from build123d import *

# Parameters (mm, degrees)
SKETCH1_W           = 170
SKETCH1_H           = 16
BOSS_EXTRUDE1_DEPTH = 2
SKETCH2_W           = 25
SKETCH2_H           = 4
CUT_EXTRUDE1_DEPTH  = 86.469292731
FILLET1_R           = 5


with BuildPart() as part:
    # Sketch1 → Boss-Extrude1 (new, symmetric)
    with BuildSketch(Plane(origin=(0, 0, 0), x_dir=(1, 0, 0), z_dir=(0, 1, 0))):
        Rectangle(SKETCH1_W, SKETCH1_H)
    extrude(amount=BOSS_EXTRUDE1_DEPTH, both=True)

    # Sketch2 → Cut-Extrude1 (cut, through all)
    with BuildSketch(Plane(origin=(0, 2, 0), x_dir=(1, 0, 0), z_dir=(0, 1, 0))):
        with Locations((47.5, 6)):
            Rectangle(SKETCH2_W, SKETCH2_H)
        with Locations((-2.5, 6)):
            Rectangle(SKETCH2_W, SKETCH2_H)
        with Locations((-52.5, 6)):
            Rectangle(SKETCH2_W, SKETCH2_H)
        with Locations((-102.5, 6)):
            Rectangle(SKETCH2_W, SKETCH2_H)
        with Locations((-152.5, 6)):
            Rectangle(SKETCH2_W, SKETCH2_H)
        with Locations((-202.5, 6)):
            Rectangle(SKETCH2_W, SKETCH2_H)
        with Locations((-252.5, 6)):
            Rectangle(SKETCH2_W, SKETCH2_H)
        with Locations((-302.5, 6)):
            Rectangle(SKETCH2_W, SKETCH2_H)
        with Locations((-352.5, 6)):
            Rectangle(SKETCH2_W, SKETCH2_H)
        with Locations((-402.5, 6)):
            Rectangle(SKETCH2_W, SKETCH2_H)
    cut_extrude1 = extrude(amount=-CUT_EXTRUDE1_DEPTH, mode=Mode.SUBTRACT)

    # Mirror1: Cut-Extrude1 across plane
    add(cut_extrude1.mirror(Plane.XY), mode=Mode.SUBTRACT)

    # Fillet1
    fillet1_edges = [part.edges().sort_by_distance(p)[0] for p in [
        (-85, 0, 8),
        (-85, 0, -8),
    ]]
    fillet(fillet1_edges, radius=FILLET1_R)


solid = part.part
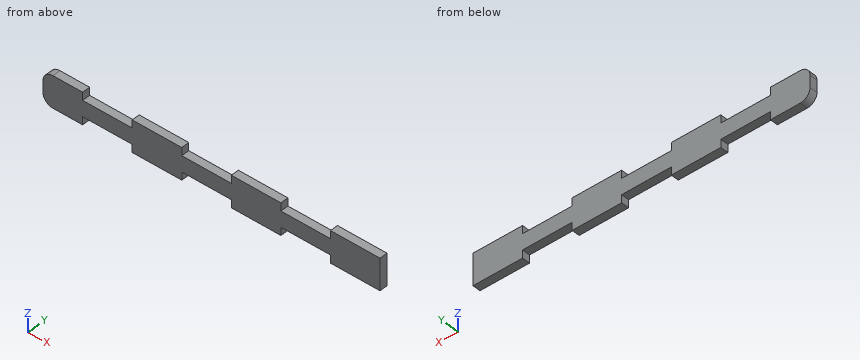
Build history of the part. All positions in model axes, mm. Round coordinates to 2 decimals unless told otherwise and drop trailing zeros. Write each loop counter-clockwise with the first axis right and the second up, starting at its lowest first coordinate (ties: lowest second). Pieces come first, ordered by that corner, then holes. Notation, with made-up numbers: (13, 20) -> (22, 20) arc R27 ccw to (22, 54) -> close; hole circle Ø9 at (41, 82.5). An arc over 180 degrees is marked (long way). Write item = value, one per line.
(1) Flat gauge pins, fed straight in: pin 1 (1.2 mm diameter, centred on x = 42.5, y = 0.5, fed in from +Z); pin 2 (2 mm diameter, centred on y = 0.5, z = -5, fed in from -X); pin 3 (1.2 mm diameter, centred on y = 0.5, z = 6.5, fed in from -X). Where does each tip first touch, or does it go through?
Answer:
pin_1 = 4
pin_2 = -84.9
pin_3 = -84.07
(2) Band-saw the part on C-C (x = -52.5). Give the cut face in (y, z).
Answer:
outline = (-2, -4) -> (2, -4) -> (2, 4) -> (-2, 4) -> close
(3) Band-saw the part on B-B (z = -5.5). Give the cut face in (x, y), then the cut area to 3 significant figures.
Answer:
outline = (-84.33, -2) -> (-65, -2) -> (-65, 2) -> (-84.33, 2) -> close; (-40, -2) -> (-15, -2) -> (-15, 2) -> (-40, 2) -> close; (10, -2) -> (35, -2) -> (35, 2) -> (10, 2) -> close; (60, -2) -> (85, -2) -> (85, 2) -> (60, 2) -> close
area = 377 mm2
(4) Probe L1, parallel to X at y = -1.05, z = -4.75; L2, parallel to X at y = -0.1, z = -5.75; L3, parallel to Z at x = 8.5, y = 0.8. List the from-to ranges inside material, lowest first.
Answer:
L1 = -84.68 to -65, -40 to -15, 10 to 35, 60 to 85
L2 = -84.18 to -65, -40 to -15, 10 to 35, 60 to 85
L3 = -4 to 4
